Check sheet for the modelled part. Datum: model origin and axes. Units: mm. A direction names the side the tool comes from. Coordinates: 2 decimals unless noted, no trailing zeros. Loops run counter-clockwise (first coordinate to the right, second up) from the corner with the lowest first, then second, coordinate; pieces in that order, holes last. Notation, with made-up numbers: M 31,83.25 L 42,83.25 A22 cw 42,118.25 Z; hole C -1.75,18 d4. An arc over 180 degrees is marked long. Use CSV: the item, a comma, the result in double quotes. Start each with the question number.
(1) Go/stop test with flat-tipped pins: pin 1 Ø12 at (x, y) = (74, -5) entering from +Z; pin 2 Ø1 at (x, y) = (-44.5, -10) entering from -Z; pin 3 Ø12 at (x, y) = (13, -5.5) entering from +Z; pin 4 Ø10 at (x, z) = (-43.5, 85.5) entering from -Y. Record where each tip stops, or that it passes through.
(2) Section check A-A on x = 0. Record the cut outline in (y, z).
(3) Set-up check for faces 1 (the conical face through (112.74, -0.49, -25.04)), 2 (the cylindrical face through (-90.6, 0.2, -33.3)): record each of +Z, -Z, +X, -X, +Y, -Y from which the full face is reachable in a straight line by a thin tool's end or side.
(4) Section check C-C on y = 6. Give the number of separate pieces and of enclosed holes in the cut face, and give its area (3 significant figures).
(5) Scan lines: line 1 (X direction, y = 11, z = -0.5); line 2 (X direction, y = -6.75, z = 0); line 3 (Z direction, x = -71, y = -1). Record each from-to range of solid material in increasing order.
(6) Draft check along X on faces 3 (the cylindrical face through (5.5, -12.46, -124.88)), 4 (the flat face through (0, 0, 24.365)), 5 (the flat face through (-26, -15, -2)). Enter one of: pulls with the +X half, pulls with the -X half, needs draft (parallel to the pull), parting line crosses it, or undercut.
(7) Section check B-B on z = 0. Record the cut outline in (x, y), and give its area (3 significant figures).
from build123d import *

# Parameters (mm, degrees)
SKETCH1_R           = 125
BOSS_EXTRUDE1_DEPTH = 15


with BuildPart() as part:
    # Sketch1 → Boss-Extrude1 (new, symmetric)
    with BuildSketch(Plane(origin=(0, 0, 0), x_dir=(1, 0, 0), z_dir=(0, 1, 0))):
        with Locations(Location((0, 0, 0), (0, 0, 270))):
            Circle(SKETCH1_R)
        with BuildLine():
            Line((34.312451849, 34.244060041), (69.217294241, 54.396380192))
            ThreePointArc((69.217294241, 54.396380192), (74.125688388, 61.706180446), (71.352549156, 70.062926922))
            ThreePointArc((71.352549156, 70.062926922), (0, 100), (-71.352549156, 70.062926922))
            ThreePointArc((-71.352549156, 70.062926922), (-74.125688388, 61.706180446), (-69.217294241, 54.396380192))
            Line((-69.217294241, 54.396380192), (-34.312451849, 34.244060041))
            ThreePointArc((-34.312451849, 34.244060041), (-31.397859232, 33.591405411), (-28.631206664, 34.716768354))
            ThreePointArc((-28.631206664, 34.716768354), (0, 45), (28.631206664, 34.716768354))
            ThreePointArc((28.631206664, 34.716768354), (31.397859232, 33.591405411), (34.312451849, 34.244060041))
        make_face(mode=Mode.SUBTRACT)
        with BuildLine():
            Line((-12.5, -46.837484988), (-12.5, -87.14212529))
            ThreePointArc((-12.5, -87.14212529), (-16.376275643, -95.04781944), (-25, -96.824583655))
            ThreePointArc((-25, -96.824583655), (-86.602540378, -50), (-96.352549156, 26.761656733))
            ThreePointArc((-96.352549156, 26.761656733), (-90.501964031, 33.341638994), (-81.717294241, 32.745745098))
            Line((-81.717294241, 32.745745098), (-46.812451849, 12.593424947))
            ThreePointArc((-46.812451849, 12.593424947), (-44.789940051, 10.395641014), (-44.381206664, 7.436968135))
            ThreePointArc((-44.381206664, 7.436968135), (-38.97114317, -22.5), (-15.75, -42.153736489))
            ThreePointArc((-15.75, -42.153736489), (-13.392080819, -43.987046425), (-12.5, -46.837484988))
        make_face(mode=Mode.SUBTRACT)
        with BuildLine():
            Line((12.5, -46.837484988), (12.5, -87.14212529))
            ThreePointArc((12.5, -87.14212529), (16.376275643, -95.04781944), (25, -96.824583655))
            ThreePointArc((25, -96.824583655), (86.602540378, -50), (96.352549156, 26.761656733))
            ThreePointArc((96.352549156, 26.761656733), (90.501964031, 33.341638994), (81.717294241, 32.745745098))
            Line((81.717294241, 32.745745098), (46.812451849, 12.593424947))
            ThreePointArc((46.812451849, 12.593424947), (44.789940051, 10.395641014), (44.381206664, 7.436968135))
            ThreePointArc((44.381206664, 7.436968135), (38.97114317, -22.5), (15.75, -42.153736489))
            ThreePointArc((15.75, -42.153736489), (13.392080819, -43.987046425), (12.5, -46.837484988))
        make_face(mode=Mode.SUBTRACT)
        with BuildLine():
            Line((-5, -19.364916731), (-5, -24.364916731))
            Line((-5, -24.364916731), (5, -24.364916731))
            Line((5, -24.364916731), (5, -19.364916731))
            ThreePointArc((5, -19.364916731), (0, 20), (-5, -19.364916731))
        make_face(mode=Mode.SUBTRACT)
    extrude(amount=BOSS_EXTRUDE1_DEPTH, both=True)

    # Sketch2 → Cut-Revolve1 (revolve, cut)
    with BuildSketch(Plane.XY, mode=Mode.PRIVATE) as cut_revolve1_sk:
        Polygon((-125, 10), (-125, -10), (-115, 0), align=None)
    revolve(cut_revolve1_sk.sketch.rotate(Axis((0, 35.426669207, 0), (0, -1, 0)), 270), axis=Axis((0, 35.426669207, 0), (0, -1, 0)), mode=Mode.SUBTRACT)


solid = part.part
Outcome:
1,pin 1,"stops at z = 103.1"
1,pin 2,"stops at z = -117"
1,pin 3,"stops at z = 124.67"
1,pin 4,"stops at y = -15"
2,outline,"M -15,-125 L -10,-125 L 0,-115 L 10,-125 L 15,-125 L 15,-100 L -15,-100 Z; M -15,-45 L 15,-45 L 15,-20 L -15,-20 Z; M -15,24.36 L 15,24.36 L 15,125 L 10,125 L 0,115 L -10,125 L -15,125 Z"
3,face 1,"none"
3,face 2,"+Y, -Y"
4,separate pieces,"1"
4,enclosed holes,"4"
4,area,"24,000 mm²"
5,line 1,"x = -125 to -100, -45 to -19.99, 19.99 to 45, 100 to 125"
5,line 2,"x = -121.75 to -100, -45 to -20, 20 to 45, 100 to 121.75"
5,line 3,"z = -91.73 to -70.42, -55.71 to -26.56, 70.42 to 91.73"
6,face 3,"parting line crosses it"
6,face 4,"undercut"
6,face 5,"needs draft"
7,outline,"M -125,-15 L -100,-15 L -100,15 L -125,15 L -125,10 L -115,0 L -125,-10 Z; M -45,-15 L -20,-15 L -20,15 L -45,15 Z; M 20,-15 L 45,-15 L 45,15 L 20,15 Z; M 100,-15 L 125,-15 L 125,-10 L 115,0 L 125,10 L 125,15 L 100,15 Z"
7,area,"2,800 mm²"
